Geometry: final body of the model. Coordinates: model frame, mm. Face numbers are marked on the shaded views. A direction names the side the tool comes from. Give positions to 0.01 mm unless a question says otherwise; leave off trailing zeros. Order: outer loops, then holes, each group sorted by start corner. A loop starts at its lowest first (then second) coordinate and runs counter-clockwise, first axis right, second up. Notation, with made-up numbers: M 39,-20.75 L 77,-20.75 A15 cw 77,-16.75 Z; hole C -38,34.5 d2. An arc over 180 degrees is marked long. Write item = value, one per line. Start each with the question number.
from build123d import *

# Parameters (mm, degrees)
SKETCH2_R           = 1.7
BOSS_EXTRUDE1_DEPTH = 3
SKETCH3_R           = 10.2
CUT_EXTRUDE1_DEPTH  = 1


with BuildPart() as part:
    # Sketch2 → Boss-Extrude1 (new body)
    # profile 1 of 7: a face of its own
    with BuildSketch(Plane.XY):
        with BuildLine():
            ThreePointArc((-17.5, 0), (-17.591670867, -1.511081774), (-17.8653389, -3))
            Line((-17.8653389, -3), (-10.5, -3))
            Line((-10.5, -3), (-10.5, 3))
            Line((-10.5, 3), (-17.8653389, 3))
            ThreePointArc((-17.8653389, 3), (-17.591670867, 1.511081774), (-17.5, 0))
        make_face()
        with Locations((-14, 0)):
            Circle(SKETCH2_R, mode=Mode.SUBTRACT)
    # profile 2 of 7: a face of its own
    with BuildSketch(Plane.XY):
        with BuildLine():
            ThreePointArc((-19.8, 0), (-20.868461247, -4.544777222), (-23.85, -8.137413594))
            Line((-23.85, -8.137413594), (-23.85, -10.882439984))
            ThreePointArc((-23.85, -10.882439984), (-20.044327099, -7.558741767), (-17.8653389, -3))
            ThreePointArc((-17.8653389, -3), (-17.591670867, -1.511081774), (-17.5, 0))
            ThreePointArc((-17.5, 0), (-17.591670867, 1.511081774), (-17.8653389, 3))
            ThreePointArc((-17.8653389, 3), (-20.044327099, 7.558741767), (-23.85, 10.882439984))
            Line((-23.85, 10.882439984), (-23.85, 8.137413594))
            ThreePointArc((-23.85, 8.137413594), (-20.868461247, 4.544777222), (-19.8, 0))
        make_face()
    # profile 3 of 7: a face of its own
    with BuildSketch(Plane.XY):
        with BuildLine():
            Line((-23.85, -10.882439984), (-23.85, -8.137413594))
            ThreePointArc((-23.85, -8.137413594), (-30, -10.2), (-36.15, -8.137413594))
            Line((-36.15, -8.137413594), (-36.15, -10.882439984))
            ThreePointArc((-36.15, -10.882439984), (-30, -12.5), (-23.85, -10.882439984))
        make_face()
    # profile 4 of 7: a face of its own
    with BuildSketch(Plane.XY):
        with BuildLine():
            Line((-36.15, -10.882439984), (-36.15, -8.137413594))
            ThreePointArc((-36.15, -8.137413594), (-40.2, 0), (-36.15, 8.137413594))
            Line((-36.15, 8.137413594), (-36.15, 10.882439984))
            ThreePointArc((-36.15, 10.882439984), (-39.955672901, 7.558741767), (-42.1346611, 3))
            ThreePointArc((-42.1346611, 3), (-42.5, 0), (-42.1346611, -3))
            ThreePointArc((-42.1346611, -3), (-39.955672901, -7.558741767), (-36.15, -10.882439984))
        make_face()
    # profile 5 of 7: a face of its own
    with BuildSketch(Plane.XY):
        with BuildLine():
            ThreePointArc((-36.15, -8.137413594), (-30, -10.2), (-23.85, -8.137413594))
            ThreePointArc((-23.85, -8.137413594), (-20.868461247, -4.544777222), (-19.8, 0))
            ThreePointArc((-19.8, 0), (-20.868461247, 4.544777222), (-23.85, 8.137413594))
            ThreePointArc((-23.85, 8.137413594), (-30, 10.2), (-36.15, 8.137413594))
            ThreePointArc((-36.15, 8.137413594), (-40.2, 0), (-36.15, -8.137413594))
        make_face()
    # profile 6 of 7: a face of its own
    with BuildSketch(Plane.XY):
        with BuildLine():
            Line((-36.15, 10.882439984), (-36.15, 8.137413594))
            ThreePointArc((-36.15, 8.137413594), (-30, 10.2), (-23.85, 8.137413594))
            Line((-23.85, 8.137413594), (-23.85, 10.882439984))
            ThreePointArc((-23.85, 10.882439984), (-30, 12.5), (-36.15, 10.882439984))
        make_face()
    # profile 7 of 7: a face of its own
    with BuildSketch(Plane.XY):
        with BuildLine():
            Line((-49.5, -3), (-42.1346611, -3))
            ThreePointArc((-42.1346611, -3), (-42.5, 0), (-42.1346611, 3))
            Line((-42.1346611, 3), (-49.5, 3))
            Line((-49.5, 3), (-49.5, -3))
        make_face()
        with Locations((-46, 0)):
            Circle(SKETCH2_R, mode=Mode.SUBTRACT)
    extrude(amount=BOSS_EXTRUDE1_DEPTH)

    # Sketch3 → Cut-Extrude1 (cut)
    with BuildSketch(Plane(origin=(0, 0, 0), x_dir=(-1, 0, 0), z_dir=(0, 0, -1))):
        with Locations((30, 0)):
            Circle(SKETCH3_R)
    extrude(amount=-CUT_EXTRUDE1_DEPTH, mode=Mode.SUBTRACT)


solid = part.part
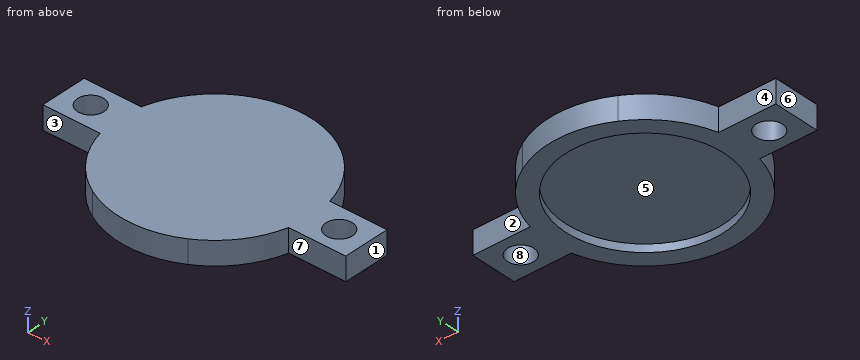
1) Ray query, L1, parallel to Y at x = -46, z = 0.4; L2, parallel to Y at x = -30, z = 0.55; L3, parallel to Y at x = -43, z = 0.2. Return the intervals inside material, ascending.
2) Cut plane A-A (x = -46). Return loops of the section in (y, z), plus the area to 3 significant figures.
3) Access query for the marked faces 1, 2, 3, 4 and 5. Directions: +Z, -Z, +X, -X, +Y, -Y. A direction counts if a zero-diameter tool reaches every point of the face in a straight line with its end or side. Return the directions, or none.
4) Draft query along Y for the marked faces 6, 7 and 8. Return one class per face: pulls with the +Y half, pulls with the -Y half, needs draft (parallel to the pull), parting line crosses it, or undercut.
5) Cut plane C-C (z = 1.7). Return loops of the section in (x, y).
6) Pin query (flat end, axial travel): pin 1 Ø0.9 at (x, z) = (-46, 1.5) entering from -Y; pin 2 Ø12 at (x, y) = (-30, 0) entering from -Z. Return the tip coordinate at first contact, or that it passes through.
7) Cut plane B-B (y = 0). Return loops of the section in (x, z), plus the area to 3 significant figures.
8) Cut plane D-D (x = -30). Return loops of the section in (y, z).
Reply:
q1.L1 = -3 to -1.7, 1.7 to 3
q1.L2 = -12.5 to -10.2, 10.2 to 12.5
q1.L3 = -3 to 3
q2.outline = M -3,0 L -1.7,0 L -1.7,3 L -3,3 Z; M 1.7,0 L 3,0 L 3,3 L 1.7,3 Z
q2.area = 7.80 mm²
q3.face_1 = +Z, -Z, +X, +Y, -Y
q3.face_2 = +Z, -Z, +X, +Y
q3.face_3 = +Z, -Z, -X, -Y
q3.face_4 = +Z, -Z, -X, +Y
q3.face_5 = -Z
q4.face_6 = needs draft
q4.face_7 = pulls with the -Y half
q4.face_8 = undercut
q5.outline = M -49.5,-3 L -42.13,-3 A12.5 ccw -17.87,-3 L -10.5,-3 L -10.5,3 L -17.87,3 A12.5 ccw -42.13,3 L -49.5,3 Z; hole C -46,0 d3.4; hole C -14,0 d3.4
q6.pin_1 = -3
q6.pin_2 = 1
q7.outline = M -49.5,0 L -47.7,0 L -47.7,3 L -49.5,3 Z; M -44.3,0 L -40.2,0 L -40.2,1 L -19.8,1 L -19.8,0 L -15.7,0 L -15.7,3 L -44.3,3 Z; M -12.3,0 L -10.5,0 L -10.5,3 L -12.3,3 Z
q7.area = 76.2 mm²
q8.outline = M -12.5,0 L -10.2,0 L -10.2,1 L 10.2,1 L 10.2,0 L 12.5,0 L 12.5,3 L -12.5,3 Z
